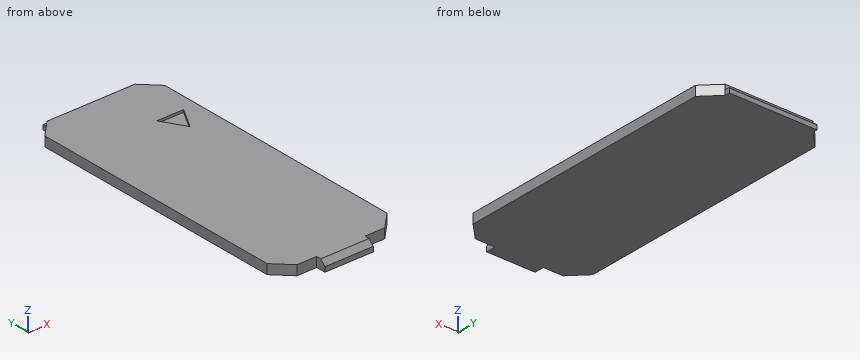
from build123d import *

# Parameters (mm, degrees)
F1_W      = 44.65
F1_H      = 108.65
F2_DEPTH  = 3.6
F3_SIZE   = 5.9976
F4_W      = 32.6548
F4_H      = 1.8
F5_DEPTH  = 1.8
F6_R      = 0.25
F7_W      = 18
F7_H      = 3.6
F8_DEPTH  = 3.6
F9_SIZE   = 1.8
F11_DEPTH = 0.9


with BuildPart() as f2:
    # F1 (on Top) → F2 (new body)
    with BuildSketch(Plane.XY):
        Rectangle(F1_W, F1_H)
    extrude(amount=F2_DEPTH)

    # F3
    f3_edges = [f2.edges().sort_by_distance(p)[0] for p in [
        (22.325, -54.325, 1.8),
        (-22.325, -54.325, 1.8),
        (-22.325, 54.325, 1.8),
        (22.325, 54.325, 1.8),
    ]]
    chamfer(f3_edges, length=F3_SIZE)

    # F4 (on face) → F5 (join)
    with BuildSketch(Plane(origin=(0, 54.325, 0), x_dir=(-1, 0, 0), z_dir=(0, 1, 0))):
        with Locations((0, 0.9)):
            Rectangle(F4_W, F4_H)
    extrude(amount=F5_DEPTH)

    # F6
    f6_edges = [f2.edges().sort_by_distance(p)[0] for p in [
        (0, 56.125, 1.8),
    ]]
    fillet(f6_edges, radius=F6_R)

    # F7 (on face) → F8 (join)
    with BuildSketch(Plane.XZ.offset(54.325)):
        with Locations((0, 1.8)):
            Rectangle(F7_W, F7_H)
    extrude(amount=F8_DEPTH)

    # F9
    f9_edges = [f2.edges().sort_by_distance(p)[0] for p in [
        (0, -57.925, 3.6),
    ]]
    chamfer(f9_edges, length=F9_SIZE)

    # F10 (on face) → F11 (cut)
    with BuildSketch(Plane.XY.offset(3.6)):
        Polygon((17.325, 34.2784180126), (7.325, 34.2784180126), (12.325, 25.6181639748), align=None)
    extrude(amount=-F11_DEPTH, mode=Mode.SUBTRACT)


solid = f2.part
Here's how the part is built. I have some questions about the finished solid (model axes, mm). Coordinates: 2 decimals unless noted, no trailing zeros. Loops run counter-clockwise (first coordinate to the right, second up) from the corner with the lowest first, then second, coordinate; pieces in that order, holes last.
1. Imagine slicing it at B-B, the plane z = 0.9. Please give me the cut outline in (x, y) (3 decimals).
2. For P1, Ø2, axis at y = 55, z = 1, coming from the +X side; P2, Ø1.2, axis at x = -3.5, y = 55, coming from the +Z side; P3, Ø1.1, axis at x = -12.5, z = 1.5, coming from the -Y side (3 decimals), each with a flat end and sliding along its axis, tell me the tip position at first contact or that it passes through.
3. Imagine slicing it at C-C, the plane x = 10.5. Please give me the cut outline in (y, z) (3 decimals).
4. Imagine slicing it at A-A, the plane x = -12.5. Please give me the cut outline in (y, z) (3 decimals).
5. Imagine slicing it at D-D, the plane x = 15. Please give me the cut outline in (y, z) (3 decimals).
6. I need wall thicknesses on L1, parallel to Y at x = 11, z = 2.05 (3 decimals); L2, parallel to Y at x = 14.5, z = 0.85 (3 decimals). Which ranges of each line are inside material? Lowest first, please.
Taken from the geometry:
1. outline: (-22.325, -48.327) - (-16.327, -54.325) - (-9, -54.325) - (-9, -57.925) - (9, -57.925) - (9, -54.325) - (16.327, -54.325) - (22.325, -48.327) - (22.325, 48.327) - (16.327, 54.325) - (16.327, 56.125) - (-16.327, 56.125) - (-16.327, 54.325) - (-22.325, 48.327) - close
2. P1: stops at x = 16.65
2. P2: stops at z = 1.8
2. P3: stops at y = -54.325
3. outline: (-54.325, 0) - (56.125, 0) - (56.125, 1.55) arc R0.25 ccw to (55.875, 1.8) - (54.325, 1.8) - (54.325, 3.6) - (34.278, 3.6) - (34.278, 2.7) - (28.779, 2.7) - (28.779, 3.6) - (-54.325, 3.6) - close
4. outline: (-54.325, 0) - (56.125, 0) - (56.125, 1.55) arc R0.25 ccw to (55.875, 1.8) - (54.325, 1.8) - (54.325, 3.6) - (-54.325, 3.6) - close
5. outline: (-54.325, 0) - (56.125, 0) - (56.125, 1.55) arc R0.25 ccw to (55.875, 1.8) - (54.325, 1.8) - (54.325, 3.6) - (34.278, 3.6) - (34.278, 2.7) - (30.251, 2.7) - (30.251, 3.6) - (-54.325, 3.6) - close
6. L1: y = -54.325 to 54.325
6. L2: y = -54.325 to 56.125
